The listing builds one solid part. Answer for the finished solid, in the listing's coordinates (mm). Face numbers are marked on the shaded views. A direction names the side the tool comes from. Coordinates: 2 decimals unless noted, no trailing zeros. Write each loop counter-clockwise with the first axis right and the second up, starting at its lowest first coordinate (ties: lowest second). Pieces come first, ordered by that corner, then holes.
Autodesk Fusion 360 part; units mm, degrees
sketch "Sketch1" plane through (0, 0, 0) normal (0, 1, 0) x (1, 0, 0)
  line L0 (-5.7502, 8.4443) -> (-5.7502, -12.9557)
  arc A0 (-5.7502, -12.9557) -> (2.2498, -12.9557) centre (-1.7502, -12.9557) ccw
  line L1 (2.2498, -12.9557) -> (2.2498, 8.4443)
  arc A1 (2.2498, 8.4443) -> (-5.7502, 8.4443) centre (-1.7502, 8.4443) ccw
  line L2 (-1.7502, 8.4443) -> (-1.7502, -12.9557) construction
  point P0 (-1.7502, 12.4443)
  point P1 (-1.7502, -16.9557)
  dimension "d1" = 29.4
  dimension "d2" = 8
extrude "Extrude1" add sketch "Sketch1" along normal blind 1
sketch "Sketch2" plane through (0, 0, 0) normal (0, -1, 0) x (1, 0, 0)
  arc A0 (-5.7502, -8.4443) -> (2.2498, -8.4443) centre (-1.7502, -8.4443) ccw
  line L0 (2.2498, -8.4443) -> (2.2498, 12.9557)
  arc A1 (2.2498, 12.9557) -> (-5.7502, 12.9557) centre (-1.7502, 12.9557) ccw
  line L1 (-5.7502, 12.9557) -> (-5.7502, -8.4443)
  arc A2 (-4.7502, -8.4443) -> (1.2498, -8.4443) centre (-1.7502, -8.4443) ccw
  line L2 (1.2498, -8.4443) -> (1.2498, 12.9557)
  arc A3 (1.2498, 12.9557) -> (-4.7502, 12.9557) centre (-1.7502, 12.9557) ccw
  line L3 (-4.7502, 12.9557) -> (-4.7502, -8.4443)
  dimension "d5" = -1
  dimension "d6" = 6
extrude "Extrude2" add sketch "Sketch2" along normal blind 2.6 contours A2 L2 A3 L3
sketch "Sketch3" plane through (0, 1, 0) normal (0, 1, 0) x (-1, 0, 0)
  arc A0 (-2.2498, -8.4443) -> (5.7502, -8.4443) centre (1.7502, -8.4443) ccw
  line L0 (5.7502, -8.4443) -> (5.7502, 12.9557)
  arc A1 (5.7502, 12.9557) -> (-2.2498, 12.9557) centre (1.7502, 12.9557) ccw
  line L1 (-2.2498, 12.9557) -> (-2.2498, -8.4443)
  line L2 (1.7502, -12.4443) -> (1.7502, 16.9557) construction
  line L3 (0.2502, 7.7557) -> (0.2502, -3.2443)
  arc A2 (0.2502, -3.2443) -> (3.2502, -3.2443) centre (1.7502, -3.2443) ccw
  line L4 (3.2502, -3.2443) -> (3.2502, 7.7557)
  arc A3 (3.2502, 7.7557) -> (0.2502, 7.7557) centre (1.7502, 7.7557) ccw
  line L5 (1.7502, 7.7557) -> (1.7502, -3.2443) construction
  line L6 (3.2502, 7.7557) -> (3.2502, 9.0057)
  line L7 (3.2502, 9.0057) -> (0.2502, 9.0057)
  line L8 (0.2502, 9.0057) -> (0.2502, 7.7557)
  circle A4 centre (1.7502, -3.2443) radius 0.85
  circle A5 centre (1.7502, -1.0443) radius 0.85
  circle A6 centre (1.7502, 1.1557) radius 0.85
  circle A7 centre (1.7502, 3.3557) radius 0.85
  circle A8 centre (1.7502, 5.5557) radius 0.85
  circle A9 centre (1.7502, 7.7557) radius 0.85
  point P0 (1.7502, 2.2557)
  point P1 (1.7502, -4.7443)
  dimension "d9" = 7
  dimension "d10" = 3
  dimension "d11" = 1.25
  dimension "d12" = 5.5
  dimension "d13" = 1.7
  dimension "d16" = 0
  dimension "d17" = 11
extrude "Extrude3" add sketch "Sketch3" along normal blind 2.2 contours L3 A2 L4 A3 L7 | A3 L7 L8 | A3 L6 L7 | A4 | A5 | A6 | A7 | A8 | A9
sketch "Sketch4" plane through (0, 1, 0) normal (0, 1, 0) x (-1, 0, 0)
  line L0 (0.2502, 9.0057) -> (3.2502, 9.0057)
  line L1 (3.2502, 9.0057) -> (3.2502, -3.2443)
  arc A0 (0.2502, -3.2443) -> (3.2502, -3.2443) centre (1.7502, -3.2443) ccw
  line L2 (0.2502, -3.2443) -> (0.2502, 9.0057)
  arc A1 (-2.2498, -8.4443) -> (5.7502, -8.4443) centre (1.7502, -8.4443) ccw
  line L3 (5.7502, -8.4443) -> (5.7502, 12.9557)
  arc A2 (5.7502, 12.9557) -> (-2.2498, 12.9557) centre (1.7502, 12.9557) ccw
  line L4 (-2.2498, 12.9557) -> (-2.2498, -8.4443)
  line L5 (4.7502, 12.9557) -> (4.7502, -8.4443)
  arc A3 (-1.2498, -8.4443) -> (4.7502, -8.4443) centre (1.7502, -8.4443) ccw
  line L6 (-1.2498, -8.4443) -> (-1.2498, 12.9557)
  arc A4 (4.7502, 12.9557) -> (-1.2498, 12.9557) centre (1.7502, 12.9557) ccw
extrude "Extrude4" add sketch "Sketch4" along normal blind 1.2 contours L5 A3 L6 A4
sketch "Sketch5" plane through (0, -2.6, 0) normal (0, -1, 0) x (1, 0, 0)
  line L0 (-4.7502, 12.9557) -> (-4.7502, -8.4443)
  arc A0 (-4.7502, -8.4443) -> (1.2498, -8.4443) centre (-1.7502, -8.4443) ccw
  line L1 (1.2498, -8.4443) -> (1.2498, 12.9557)
  arc A1 (1.2498, 12.9557) -> (-4.7502, 12.9557) centre (-1.7502, 12.9557) ccw
  line L2 (-0.2502, 9.0057) -> (-0.2502, -3.2443)
  arc A2 (-3.2502, -3.2443) -> (-0.2502, -3.2443) centre (-1.7502, -3.2443) ccw
  line L3 (-3.2502, -3.2443) -> (-3.2502, 9.0057)
  line L4 (-3.2502, 9.0057) -> (-0.2502, 9.0057)
  circle A3 centre (-1.7502, 7.7557) radius 0.5455
  circle A4 centre (-1.7502, 5.5557) radius 0.5
  circle A5 centre (-1.7502, 3.3557) radius 0.5
  circle A6 centre (-1.7502, 1.1557) radius 0.5
  circle A7 centre (-1.7502, -1.0443) radius 0.5
  circle A8 centre (-1.7502, -3.2443) radius 0.5
  dimension "d22" = 1
extrude "Extrude5" add sketch "Sketch5" along normal blind 1.5 contours A3 | A4 | A5 | A6 | A7 | A8
sketch "Sketch6" plane through (0, 3.2, 0) normal (0, 1, 0) x (-1, 0, 0)
  line L0 (0.2502, 9.0057) -> (0.2502, -3.2443)
  arc A0 (0.2502, -3.2443) -> (3.2502, -3.2443) centre (1.7502, -3.2443) ccw
  line L1 (3.2502, -3.2443) -> (3.2502, 9.0057)
  line L2 (3.2502, 9.0057) -> (0.2502, 9.0057)
  circle A1 centre (1.7502, 7.7557) radius 0.85
  line L3 (0.9002, 7.7557) -> (2.6002, 7.7557)
  point P0 (1.7502, 7.7557)
ref_plane "WorkPlane1" through (-1.7502, 3.2, 7.7557) normal (0, 0, 1) x (-1, 0, 0)
sketch "Sketch7" plane through (-1.7502, 3.2, 7.7557) normal (0, 0, 1) x (1, 0, 0)
  circle A0 centre (0, 1.2359) radius 1.5
  line L0 (1.5, 1.2359) -> (-1.5, 1.2359)
  point P0 (-0.85, 0)
  point P1 (0.85, 0)
  dimension "d26" = 3
revolve "Revolve1" cut sketch "Sketch7" angle 360 about axis through (-0.2502, 4.4359, 7.7557) along (-1, 0, 0) contours A0 L0 picked at (-0.3665, 0.8958)
pattern_linear "R-Pattern1" count 6 spacing 2.2 along (0, 0, -1) of "Revolve1"
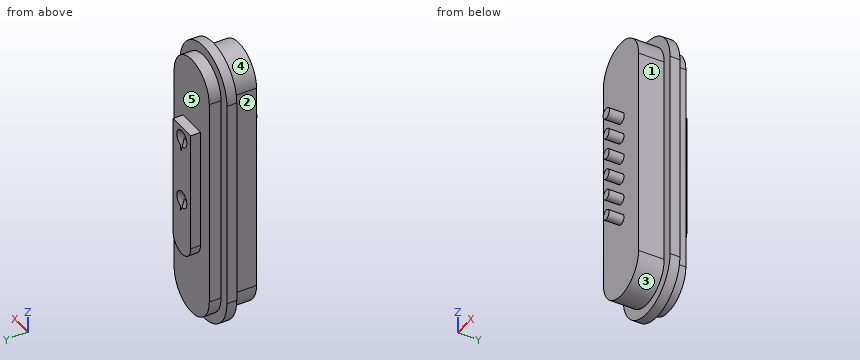
1. Flat-ended cylindrical pins translate along their axes: P1, Ø0.5, axis at y = 2.5, z = 2, coming from the -X side; P2, Ø2, axis at x = -0.5, y = -1.5, coming from the -Z side; P3, Ø0.8, axis at y = 2.5, z = 1.5, coming from the +X side. Find the tip coordinate at first contact, or state that the pin passes through.
Results found:
P1: stops at x = -3.25
P2: stops at z = -11.43
P3: stops at x = 1.25
2. For a pull along Z with two mould halves and no side action, classify the marked faces 3, 4 and 5 as pulls with the +Z half, pulls with the -Z half, needs draft (parallel to the pull), parting line crosses it, or undercut.
Results found:
face 3: pulls with the -Z half
face 4: pulls with the +Z half
face 5: needs draft
3. Section C-C on x = -4.25 is taken. Give the vertices of the cut face in (y, z).
Results found:
outline: (-2.6, -10.1) - (0, -10.1) - (0, -11.57) - (1, -11.57) - (1, -10.1) - (2.2, -10.1) - (2.2, 14.61) - (1, 14.61) - (1, 16.08) - (0, 16.08) - (0, 14.61) - (-2.6, 14.61) - close
4. Section A-A on z = 2.5 is taken. Give the vertices of the cut face in (x, y), then the cut area to 3 significant figures.
Results found:
outline: (-5.75, 0) - (-4.75, 0) - (-4.75, -2.6) - (1.25, -2.6) - (1.25, 0) - (2.25, 0) - (2.25, 1) - (1.25, 1) - (1.25, 2.2) - (-0.25, 2.2) - (-0.25, 3.2) - (-3.25, 3.2) - (-3.25, 2.2) - (-4.75, 2.2) - (-4.75, 1) - (-5.75, 1) - close
area: 33.8 mm2
5. Section D-D on y = -0.5 is taken. Give the vertices of the cut face in (x, z).
Results found:
outline: (-4.75, -8.44) arc R3 ccw to (1.25, -8.44) - (1.25, 12.96) arc R3 ccw to (-4.75, 12.96) - close
6. Section B-B on y = -3.5 is taken. Give the vertices of the cut face in (x, z).
Results found:
outline: circle Ø1.09 at (-1.75, 7.76); circle Ø1 at (-1.75, -3.24); circle Ø1 at (-1.75, -1.04); circle Ø1 at (-1.75, 1.16); circle Ø1 at (-1.75, 3.36); circle Ø1 at (-1.75, 5.56)
7. Find the intervals of material crossed by L1, parallel to Y at x = -4.75, z = -10.75; L2, parallel to Y at x = 1, z = 8, in increasing order.
Results found:
L1: y = 0 to 1
L2: y = -2.6 to 2.2
8. A tool of negligible diameter and unlimited length cuts with its end or side. For the marked faces 1 and 2, from which of +Z, -Z, +X, -X, +Y, -Y can it reach the whole face along a straight path? Write none if from no direction.
Results found:
face 1: +Z, -Z, +X, -Y
face 2: +Z, -Z, -X, -Y
